```python
from build123d import *

# Parameters (mm, degrees)
F1_DEPTH = 12.7
F3_D     = 7.5946
F5_DEPTH = 25.4


with BuildPart() as f1:
    # F0 (on Front) → F1 (new body)
    with BuildSketch(Plane.XZ):
        Polygon((-29.167796, -5.559607), (-24.333354, 0), (3.545257, 0), (11.763807, -8.782567), (18.78079, -20.983703), (21.036864, -25.818144), (22.326047, -25.818144), (27.099216, -19.453921), (21.389281, -7.218347), (7.573958, 6.526496), (-28.523203, 6.526496), (-36.271484, -6.691031), (-31.504442, -10.2329), align=None)
    extrude(amount=F1_DEPTH)

    # F3 (through all)
    with Locations(Plane.XZ.offset(12.7)):
        with Locations((20.701887, -15.946049)):
            Hole(F3_D / 2)

    # F4 (on face) → F5 (cut)
    with BuildSketch(Plane.XZ.offset(12.7)):
        with BuildLine():
            ThreePointArc((26.33537, -17.817108), (23.104833, -20.704799), (18.78079, -20.983703))
            Line((18.78079, -20.983703), (21.036864, -25.818144))
            Line((21.036864, -25.818144), (22.326047, -25.818144))
            Line((22.326047, -25.818144), (27.099216, -19.453921))
            Line((27.099216, -19.453921), (26.33537, -17.817108))
        make_face()
    extrude(amount=-F5_DEPTH, mode=Mode.SUBTRACT)


solid = f1.part
```
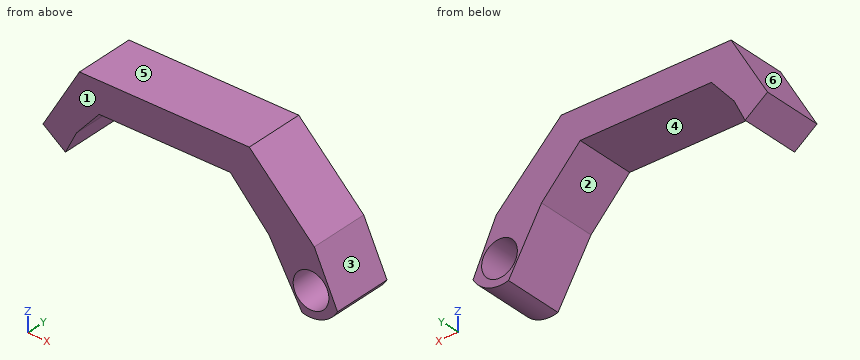
Check sheet for the modelled part. Datum: model origin and axes. Units: mm. Face numbers are marked on the shaded views. A direction names the side the tool comes from. Round coordinates to 2 decimals unless told otherwise and drop trailing zeros. Write each loop counter-clockwise with the first axis right and the second up, starting at its lowest first coordinate (ties: lowest second). Pieces come first, ordered by that corner, then holes. Notation, with made-up numbers: (-29.75, 42) -> (10.25, 42) arc R24 cw to (10.25, 73) -> close; hole circle Ø2 at (28, 76). An arc over 180 degrees is marked (long way). One line per question, with ' | ' between items. Start each with the question number.
1. Sectioned sample at D-D, the plane z = -19. Record the cut outline in (x, y), then the cut area to 3 significant figures.
2. Release check for a two-part mould opening along X. For the marked faces 3, 4, 5 and 6 record: +X half, -X half, draft (parallel to the pull), parting line (faces both ways), or undercut.
3. Scan lines: line 1 along Z through (x, y) = (-3.5, -3); line 2 along Z through (x, y) = (23.5, -10.75); line 3 along X through (y, z) = (-10.5, -16.5). Record each from-to range of solid material in increasing order. Write a range as from..to.
4. Sectioned sample at B-B, the plane y = -10.75. Record the cut outline in (x, z), then the cut area to 3 significant figures.
5. Sectioned sample at A-A, the plane z = -2.25. Record the cut outline in (x, y), then the cut area to 3 significant figures.
6. Sectioned sample at C-C, the plane x = -12. Record the cut outline in (y, z), then the cut area to 3 significant figures.
7. Set-up check for the marked faces 1 and 2: record each of +Z, -Z, +X, -X, +Y, -Y from which the full face is reachable in a straight line by a thin tool's end or side.
8. Depth check by flat-ended pin: pin 1 (1 mm diameter, centred on y = -2.5, z = -15.5, fed in from +X); pin 2 (1.5 mm diameter, centred on y = -6, z = -3, fed in from +X); pin 3 (1 mm diameter, centred on y = -9, z = -2, fed in from +X); pin 4 (4.5 mm diameter, centred on x = 20.7, z = -15.95, fed in from -Y). Enter the tip coordinate at first touch or a pass-through.
Taken from the geometry:
1) outline: (17.64, -12.7) -> (18.45, -12.7) -> (18.45, 0) -> (17.64, 0) -> close; (22.96, -12.7) -> (25.49, -12.7) -> (25.49, 0) -> (22.96, 0) -> close | area: 42.4 mm^2
2) face 3: +X half | face 4: undercut | face 5: draft | face 6: -X half
3) line 1: z = 0..6.53 | line 2: z = -20.52..-18.51, -13.38..-11.74 | line 3: x = 16.2..16.95, 24.46..25.72
4) outline: (-36.27, -6.69) -> (-31.5, -10.23) -> (-29.17, -5.56) -> (-24.33, 0) -> (3.55, 0) -> (11.76, -8.78) -> (18.78, -20.98) arc R6.64 ccw to (26.34, -17.82) -> (21.39, -7.22) -> (7.57, 6.53) -> (-28.52, 6.53) -> close; hole circle Ø7.59 at (20.7, -15.95) | area: 490 mm^2
5) outline: (-33.67, -12.7) -> (-26.29, -12.7) -> (-26.29, 0) -> (-33.67, 0) -> close; (5.65, -12.7) -> (16.4, -12.7) -> (16.4, 0) -> (5.65, 0) -> close | area: 230 mm^2
6) outline: (-12.7, 0) -> (0, 0) -> (0, 6.53) -> (-12.7, 6.53) -> close | area: 82.9 mm^2
7) face 1: +Z, -Z, +X, -X, -Y | face 2: -Z, +Y, -Y
8) pin 1: stops at x = 25.49 | pin 2: stops at x = 17.9 | pin 3: stops at x = 16.65 | pin 4: passes through
